Geometry: final body of the model. Coordinates: model frame, mm. Face numbers are marked on the shaded views. Give positions to 0.01 mm unless a question says otherwise; leave off trailing zeros. Order: outer loops, then holes, each group sorted by start corner. A loop starts at its lowest first (then second) coordinate and runs counter-clockwise, first axis right, second up. Notation, with made-up numbers: (11, 83.5) -> (16, 83.5) arc R34 cw to (16, 117.5) -> close; hole circle Ø11 at (-27.75, 19). An arc over 180 degrees is marked (long way). One line per question, with ' | ' between items. Start each with the question number.
(1) Mould query, pull axis X, two halves, no side actions, for the marked faces 1, 2 and 3. Classes: +X half, -X half, draft (parallel to the pull), parting line (faces both ways), or undercut.
(2) Section C-C (x = 40). Return loops of the section in (y, z).
(3) Ray query, L1, parallel to Y at x = 21, z = -9.5; L2, parallel to Z at x = -56.5, y = 47; L3, parallel to Z at x = 116.5, y = 23.5. Return the intervals inside material, ascending.
(4) Section A-A (x = 73.5). Return loops of the section in (y, z).
(5) Section D-D (y = 101). Return loops of the section in (x, z), then the cut area to 3 significant figures.
(6) First-contact query: pin 1 Ø2 at (x, y) = (47.5, 66) entering from +Z; pin 2 Ø3 at (x, y) = (-34, 45) entering from -Z; pin 3 Ø19.5 at (y, z) = (63.5, -11) entering from +X; pin 4 Ø19 at (x, z) = (135, -25.5) entering from -Y. Flat tips, straight axial feed; report the tip coordinate or a pass-through.
(7) Section B-B (y = 12.5). Return loops of the section in (x, z).
```python
from build123d import *

# Parameters (mm, degrees)
BOSS_EXTRUDE1_DEPTH = 101.6
BOSS_EXTRUDE2_START = -33.02
BOSS_EXTRUDE2_DEPTH = 25.4
SKETCH4_W           = 195.058436962
SKETCH4_H           = 25.4
CUT_EXTRUDE1_DEPTH  = 38.1
SKETCH5_W           = 191.898505545
SKETCH5_H           = 25.4
CUT_EXTRUDE4_DEPTH  = 38.1
CUT_EXTRUDE5_DEPTH  = 101.6
BOSS_EXTRUDE3_START = -63.5
BOSS_EXTRUDE3_DEPTH = 25.4
FILLET1_R           = 10.16
FILLET2_R           = 10.16
FILLET3_R           = 10.16
FILLET4_R           = 10.16
SKETCH9_W           = 22.86
SKETCH9_H           = 17.78
CUT_EXTRUDE6_DEPTH  = 50.8
SKETCH10_W          = 7.656009699
SKETCH10_H          = 32.499666645
CUT_EXTRUDE7_DEPTH  = 77.2
CUT_EXTRUDE8_DEPTH  = 77.2
SKETCH12_W          = 32.499666645
SKETCH12_H          = 7.62
CUT_EXTRUDE9_DEPTH  = 50.8
FILLET6_R           = 5.08


with BuildPart() as part:
    # Sketch1 → Boss-Extrude1 (new body)
    with BuildSketch(Plane.XY):
        Polygon((0, 0), (-69.85, 0), (-69.85, 46.373441022), (-22.065879406, 76.2), (184.15, 76.2), (184.15, 0), align=None)
    extrude(amount=-BOSS_EXTRUDE1_DEPTH)

    # Sketch3 → Boss-Extrude2 (add)
    with BuildSketch(Plane(origin=(0, 76.2, 0), x_dir=(1, 0, 0), z_dir=(0, 1, 0)).offset(BOSS_EXTRUDE2_START)):
        Polygon((-45.019314853, 101.6), (25.443042364, 319.069575379), (61.864542757, 307.268638321), (-4.774190667, 101.6), align=None)
        Polygon((-4.774190667, 0), (-45.019314853, 0), (25.443042364, -217.469575379), (61.864542757, -205.668638321), align=None)
    extrude(amount=-BOSS_EXTRUDE2_DEPTH)

    # Sketch4 → Cut-Extrude1 (cut)
    with BuildSketch(Plane.XY):
        with Locations((92.755027814, 30.48)):
            Rectangle(SKETCH4_W, SKETCH4_H)
    extrude(amount=-CUT_EXTRUDE1_DEPTH, mode=Mode.SUBTRACT)

    # Sketch5 → Cut-Extrude4 (cut)
    with BuildSketch(Plane(origin=(0, 0, -101.6), x_dir=(-1, 0, 0), z_dir=(0, 0, -1))):
        with Locations((-91.175062106, 30.48)):
            Rectangle(SKETCH5_W, SKETCH5_H)
    extrude(amount=-CUT_EXTRUDE4_DEPTH, mode=Mode.SUBTRACT)

    # Sketch6 → Cut-Extrude5 (cut)
    with BuildSketch(Plane(origin=(0, 76.2, 0), x_dir=(1, 0, 0), z_dir=(0, 1, 0))):
        Polygon((28.659266364, 0), (51.128382236, 22.86), (152.752463445, 22.86), (152.752463445, 0), align=None)
        Polygon((152.752463445, 78.74), (152.752463445, 101.6), (28.659266364, 101.6), (51.128382236, 78.74), align=None)
    extrude(amount=-CUT_EXTRUDE5_DEPTH, mode=Mode.SUBTRACT)

    # Sketch8 → Boss-Extrude3 (add)
    with BuildSketch(Plane.XY.offset(BOSS_EXTRUDE3_START)):
        Polygon((184.15, 76.2), (184.15, 114.315616278), (165.003698403, 114.315616278), (137.329725858, 76.2), align=None)
    extrude(amount=BOSS_EXTRUDE3_DEPTH)

    # Fillet1
    fillet1_edges = [part.edges().sort_by_distance(p)[0] for p in [
        (-9.788136245, 43.18, 108.734787689),
    ]]
    fillet(fillet1_edges, radius=FILLET1_R)

    # Fillet2
    fillet2_edges = [part.edges().sort_by_distance(p)[0] for p in [
        (-9.788136245, 17.78, 108.734787689),
    ]]
    fillet(fillet2_edges, radius=FILLET2_R)

    # Fillet3
    fillet3_edges = [part.edges().sort_by_distance(p)[0] for p in [
        (-9.788136245, 43.18, -210.334787689),
    ]]
    fillet(fillet3_edges, radius=FILLET3_R)

    # Fillet4
    fillet4_edges = [part.edges().sort_by_distance(p)[0] for p in [
        (-9.788136245, 17.78, -210.334787689),
    ]]
    fillet(fillet4_edges, radius=FILLET4_R)

    # Sketch9 → Cut-Extrude6 (cut)
    with BuildSketch(Plane(origin=(184.15, 0, 0), x_dir=(0, 0, -1), z_dir=(1, 0, 0))):
        with Locations((90.17, 8.89)):
            Rectangle(SKETCH9_W, SKETCH9_H)
        with Locations((11.43, 8.89)):
            Rectangle(SKETCH9_W, SKETCH9_H)
    extrude(amount=-CUT_EXTRUDE6_DEPTH, mode=Mode.SUBTRACT)

    # Sketch10 → Cut-Extrude7 (cut, through all)
    with BuildSketch(Plane(origin=(0, 76.2, 0), x_dir=(1, 0, 0), z_dir=(0, 1, 0))):
        with Locations((180.321995151, 16.249833323)):
            Rectangle(SKETCH10_W, SKETCH10_H)
        with Locations((180.321995151, 85.350166677)):
            Rectangle(SKETCH10_W, SKETCH10_H)
    extrude(amount=-CUT_EXTRUDE7_DEPTH, mode=Mode.SUBTRACT)

    # Sketch11 → Cut-Extrude8 (cut, through all)
    with BuildSketch(Plane(origin=(0, 76.2, 0), x_dir=(1, 0, 0), z_dir=(0, 1, 0))):
        Polygon((152.752463445, 22.86), (152.752463445, 32.499666645), (60.768048881, 32.499666645), (51.128382236, 22.86), align=None)
        Polygon((152.752463445, 78.74), (152.752463445, 69.100333355), (60.768048881, 69.100333355), (51.128382236, 78.74), align=None)
    extrude(amount=-CUT_EXTRUDE8_DEPTH, mode=Mode.SUBTRACT)

    # Sketch12 → Cut-Extrude9 (cut)
    with BuildSketch(Plane(origin=(176.493990301, 0, 0), x_dir=(0, 0, -1), z_dir=(1, 0, 0))):
        with Locations((85.350166677, 72.39)):
            Rectangle(SKETCH12_W, SKETCH12_H)
        with Locations((85.350166677, 46.99)):
            Rectangle(SKETCH12_W, SKETCH12_H)
        with Locations((16.249833323, 46.99)):
            Rectangle(SKETCH12_W, SKETCH12_H)
        with Locations((16.249833323, 72.39)):
            Rectangle(SKETCH12_W, SKETCH12_H)
    extrude(amount=-CUT_EXTRUDE9_DEPTH, mode=Mode.SUBTRACT)

    # Fillet6
    fillet6_edges = [part.edges().sort_by_distance(p)[0] for p in [
        (152.752463445, 68.58, -16.249833323),
        (152.752463445, 50.8, -16.249833323),
        (152.752463445, 50.8, -85.350166677),
        (152.752463445, 68.58, -85.350166677),
    ]]
    fillet(fillet6_edges, radius=FILLET6_R)


solid = part.part
```
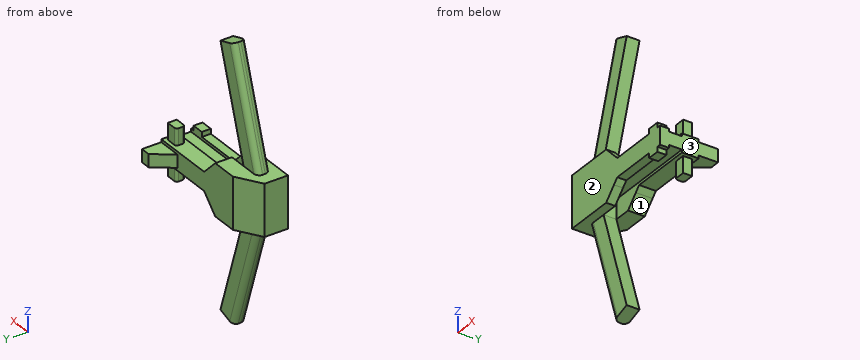
Response:
1) face 1: undercut | face 2: draft | face 3: +X half
2) outline: (0, -90.06) -> (17.78, -90.06) -> (17.78, -63.5) -> (43.18, -63.5) -> (43.18, -90.06) -> (76.2, -90.06) -> (76.2, -11.54) -> (43.18, -11.54) -> (43.18, -38.1) -> (17.78, -38.1) -> (17.78, -11.54) -> (0, -11.54) -> close; (17.78, -314.35) -> (43.18, -314.35) -> (43.18, -239.79) -> (17.78, -239.79) -> close; (17.78, 138.19) -> (43.18, 138.19) -> (43.18, 212.75) -> (17.78, 212.75) -> close
3) L1: y = 0 to 17.78, 43.18 to 76.2 | L2: z = -101.6 to 0 | L3: z = -63.5 to -38.1
4) outline: (0, -69.1) -> (17.78, -69.1) -> (17.78, -63.5) -> (43.18, -63.5) -> (43.18, -69.1) -> (76.2, -69.1) -> (76.2, -32.5) -> (43.18, -32.5) -> (43.18, -38.1) -> (17.78, -38.1) -> (17.78, -32.5) -> (0, -32.5) -> close
5) outline: (155.34, -63.5) -> (184.15, -63.5) -> (184.15, -38.1) -> (155.34, -38.1) -> close | area: 732 mm^2
6) pin 1: stops at z = -18.15 | pin 2: stops at z = -101.6 | pin 3: stops at x = 176.49 | pin 4: stops at y = 0
7) outline: (-69.85, -101.6) -> (28.66, -101.6) -> (51.13, -78.74) -> (60.77, -69.1) -> (152.75, -69.1) -> (152.75, -78.74) -> (176.49, -78.74) -> (176.49, -69.1) -> (184.15, -69.1) -> (184.15, -32.5) -> (176.49, -32.5) -> (176.49, -22.86) -> (152.75, -22.86) -> (152.75, -32.5) -> (60.77, -32.5) -> (51.13, -22.86) -> (28.66, 0) -> (-69.85, 0) -> close
